```python
from build123d import *

# Parameters (mm, degrees)
ESQUISSE1_W             = 15
ESQUISSE1_H             = 83
BOSS_EXTRU_1_DEPTH      = 6
ESQUISSE2_R             = 11
BOSS_EXTRU_2_DEPTH      = 6
ESQUISSE4_R             = 1.65
ESQUISSE4_R_2           = 1.005
ESQUISSE4_R_3           = 6.45
ENL_V_MAT_EXTRU_2_DEPTH = 10
ESQUISSE5_R             = 3
ESQUISSE5_R_2           = 2
ENL_V_MAT_EXTRU_3_DEPTH = 3


with BuildPart() as part:
    # Esquisse1 → Boss.-Extru.1 (new body)
    with BuildSketch(Plane.XY):
        with Locations((7.5, 41.5)):
            Rectangle(ESQUISSE1_W, ESQUISSE1_H)
    extrude(amount=BOSS_EXTRU_1_DEPTH)

    # Esquisse2 → Boss.-Extru.2 (add)
    with BuildSketch(Plane.XY.offset(6)):
        with Locations((7.5, 7.5)):
            Circle(ESQUISSE2_R)
        with Locations((7.5, 75.5)):
            Circle(ESQUISSE2_R)
    extrude(amount=-BOSS_EXTRU_2_DEPTH)

    # Esquisse4 → Enlèv. mat.-Extru.2 (cut)
    with BuildSketch(Plane(origin=(0, 0, 0), x_dir=(-1, 0, 0), z_dir=(0, 0, -1))):
        with Locations((-7.5, 75.5)):
            Circle(ESQUISSE4_R)
        with Locations((-7.5, 67.5)):
            Circle(ESQUISSE4_R_2)
        with Locations((-15.5, 75.5)):
            Circle(ESQUISSE4_R_2)
        with Locations((-7.5, 83.5)):
            Circle(ESQUISSE4_R_2)
        with Locations((0.5, 75.5)):
            Circle(ESQUISSE4_R_2)
        with Locations((-7.5, 7.5)):
            Circle(ESQUISSE4_R_3)
    extrude(amount=-ENL_V_MAT_EXTRU_2_DEPTH, mode=Mode.SUBTRACT)

    # Esquisse5 → Enlèv. mat.-Extru.3 (cut)
    with BuildSketch(Plane(origin=(0, 0, 0), x_dir=(-1, 0, 0), z_dir=(0, 0, -1))):
        with Locations((-7.5, 75.5)):
            Circle(ESQUISSE5_R)
        with Locations((-15.5, 75.5)):
            Circle(ESQUISSE5_R_2)
        with Locations((-7.5, 83.5)):
            Circle(ESQUISSE5_R_2)
        with Locations((0.5, 75.5)):
            Circle(ESQUISSE5_R_2)
        with Locations((-7.5, 67.5)):
            Circle(ESQUISSE5_R_2)
    extrude(amount=-ENL_V_MAT_EXTRU_3_DEPTH, mode=Mode.SUBTRACT)


solid = part.part
```
CAD build for the part. Positions are in the model's coordinates, mm. A direction names the side the tool comes from. Round coordinates to 2 decimals unless told otherwise and drop trailing zeros. Loops run counter-clockwise (first coordinate to the right, second up) from the corner with the lowest first, then second, coordinate; pieces in that order, holes last. Notation, with made-up numbers: M 48.25,55 L 64.25,55 A17 cw 64.25,88 Z; hole C 26.25,-20.5 d3. An arc over 180 degrees is marked long. Return JSON: item names as keys, results as strings. Group by question number.
(1) Saw through at C-C, the plane x = 7.5. Give the number of separate pieces and of enclosed holes in the cut face, and give its area (3 significant figures).
(2) Wall check: probe 1 along Y at (x, z) = (7.5, 2.1); probe 2 along Y at (x, z) = (7.5, 4.55) (3 decimals); probe 3 along X at (y, z) = (75.5, 4.8) (3 decimals). Give the ranges that are in metal, low to high. Write a range as [from, to].
(3) Drop flat-ended pins along their axis: P1, Ø2, axis at x = 8, y = 68, coming from the -Z side; P2, Ø3, axis at y = 54.5, z = 2, coming from the +X side; P3, Ø1.8, axis at y = 36, z = 2, coming from the -X side. Give the stop position or say it passes through.
(4) Saw through at B-B, the plane y = 75.5. List the corners of the cut face in (x, z) (3 decimals), and give its area (3 significant figures).
(5) Saw through at D-D, the plane x = 11.5. List the corners of the cut face in (y, z).
(6) Saw through at A-A, the plane z = 4. List the corners of the cut face in (x, y) (3 decimals), and give its area (3 significant figures).
(7) Mould opens along Y. For faces 4 (the flat face through (0, 41, 3)), 5 (the flat face through (7, 42, 0)) say: +Y half, -Y half, draft (parallel to the pull), parting line (faces both ways), or undercut.
(8) Tool access for faces 1 (the flat face through (-1.4, 74.6, 3)), 2 (the cylindrical face through (7.715, 77.136, 4.479)), 3 (the flat face through (15, 41, 3)): list every direction of +Z, -Z, +X, -X, +Y, -Y with a clear straight run to the whole face (end or side of a thin tool).
Answer list:
{
 "1": {"separate pieces": "5", "enclosed holes": "0", "area": "399 mm2"},
 "2": {"probe 1": "[-3.5, 1.05], [13.95, 65.5], [69.5, 72.5], [78.5, 81.5], [85.5, 86.5]", "probe 2": "[-3.5, 1.05], [13.95, 66.495], [68.505, 73.85], [77.15, 82.495], [84.505, 86.5]", "probe 3": "[-3.5, -1.505], [0.505, 5.85], [9.15, 14.495], [16.505, 18.5]"},
 "3": {"P1": "z = 3", "P2": "x = 15", "P3": "x = 0"},
 "4": {"outline": "M -3.5,0 L -2.5,0 L -2.5,3 L -1.505,3 L -1.505,6 L -3.5,6 Z; M 0.505,3 L 1.5,3 L 1.5,0 L 4.5,0 L 4.5,3 L 5.85,3 L 5.85,6 L 0.505,6 Z; M 9.15,3 L 10.5,3 L 10.5,0 L 13.5,0 L 13.5,3 L 14.495,3 L 14.495,6 L 9.15,6 Z; M 16.505,3 L 17.5,3 L 17.5,0 L 18.5,0 L 18.5,6 L 16.505,6 Z", "area": "68.0 mm2"},
 "5": {"outline": "M -2.75,0 L 2.44,0 L 2.44,6 L -2.75,6 Z; M 12.56,0 L 85.75,0 L 85.75,6 L 12.56,6 Z"},
 "6": {"outline": "M 0,15.547 A11 ccw long 15,15.547 L 15,67.453 A11 ccw long 0,67.453 Z; hole C -0.5,75.5 d2.01; hole C 7.5,7.5 d12.9; hole C 7.5,75.5 d3.3; hole C 7.5,67.5 d2.01; hole C 7.5,83.5 d2.01; hole C 15.5,75.5 d2.01", "area": "1,330 mm2"},
 "7": {"face 4": "undercut", "face 5": "draft"},
 "8": {"face 1": "-Z", "face 2": "+Z, -Z", "face 3": "+Z, -Z, +X"}
}
